Verification items for the finished model (mm, model axes). A direction names the side the tool comes from. Give positions to 0.01 mm unless a question says otherwise; leave off trailing zeros. Loops run counter-clockwise (first coordinate to the right, second up) from the corner with the lowest first, then second, coordinate; pieces in that order, holes last. Notation, with made-up numbers: M 45.5,53.25 L 81.5,53.25 A25 ccw 81.5,92.25 Z; hole C 46,61.5 d9. An arc over 180 degrees is marked long. Answer in a Markdown table with one row per item.
```python
from build123d import *

# Parameters (mm, degrees)
F0_W     = 45
F0_H     = 45
F1_DEPTH = 36
F2_T     = -2
F3_W     = 30
F3_H     = 30
F4_DEPTH = 25


with BuildPart() as f1:
    # F0 (on Front) → F1 (new body)
    with BuildSketch(Plane.XZ):
        Rectangle(F0_W, F0_H)
    extrude(amount=F1_DEPTH)

    # F2
    f2_openings = [f1.faces().sort_by_distance(p)[0] for p in [
        (0, -36, 0),
    ]]
    offset(amount=F2_T, openings=f2_openings)

    # F3 (on face) → F4 (cut)
    with BuildSketch(Plane(origin=(0, 0, 0), x_dir=(-1, 0, 0), z_dir=(0, 1, 0))):
        Rectangle(F3_W, F3_H)
    extrude(amount=-F4_DEPTH, mode=Mode.SUBTRACT)


solid = f1.part
```
Item 1: Sectioned sample at D-D (z = 19.5). Record the cut outline in (x, y).
Reported:
| item | result |
|---|---|
| outline | M -22.5,-36 L -20.5,-36 L -20.5,-2 L 20.5,-2 L 20.5,-36 L 22.5,-36 L 22.5,0 L -22.5,0 Z |
Item 2: Tool access check on faces 1 (the flat face through (0, -1, -15)), 2 (the flat face through (0, -19, -20.5)), 3 (the flat face through (-0.3, 0, 15.3)). Record the directions out of +Z, -Z, +X, -X, +Y, -Y that give a thin tool (end or side, any length) a straight path to the whole face; none if there is none.
Reported:
| item | result |
|---|---|
| face 1 | +Y, -Y |
| face 2 | -Y |
| face 3 | +Z, -Z, +X, -X, +Y |
Item 3: Sectioned sample at C-C (y = -8). Record the cut outline in (x, z).
Reported:
| item | result |
|---|---|
| outline | M -22.5,-22.5 L 22.5,-22.5 L 22.5,22.5 L -22.5,22.5 Z; hole M -20.5,-20.5 L 20.5,-20.5 L 20.5,20.5 L -20.5,20.5 Z |
Item 4: Sectioned sample at A-A (z = -13.5). Record the cut outline in (x, y), and give its area (3 significant figures).
Reported:
| item | result |
|---|---|
| outline | M -22.5,-36 L -20.5,-36 L -20.5,-2 L -15,-2 L -15,0 L -22.5,0 Z; M 15,-2 L 20.5,-2 L 20.5,-36 L 22.5,-36 L 22.5,0 L 15,0 Z |
| area | 166 mm^2 |
Item 5: Scan lines: L1, parallel to X at y = -12, z = -19; L2, parallel to Y at x = 14.5, z = 15.5. Record each from-to range of solid material in increasing order. Write a range as [from, to].
Reported:
| item | result |
|---|---|
| L1 | x = [-22.5, -20.5], [20.5, 22.5] |
| L2 | y = [-2, 0] |
Item 6: Release check for a two-part mould opening along Z. For faces 4 (the flat face through (22.5, -18, 0)), 5 (the flat face through (0, -18, -22.5)), 6 (the flat face through (-20.5, -19, 0)) record: released by +Z, released by -Z, zero draft, split by the parting line, or undercut.
Reported:
| item | result |
|---|---|
| face 4 | zero draft |
| face 5 | released by -Z |
| face 6 | undercut |
Item 7: Go/stop test with a flat-tipped pin: pin 1 (4 mm diameter, centred on x = -6, z = -16.5, fed in from -Y). Record where the tip stops, or that it passes through.
Reported:
| item | result |
|---|---|
| pin 1 | stops at y = -2 |
Item 8: Sectioned sample at B-B (x = -0.5). Record the cut outline in (y, z), and give its area (3 significant figures).
Reported:
| item | result |
|---|---|
| outline | M -36,-22.5 L 0,-22.5 L 0,-15 L -2,-15 L -2,-20.5 L -36,-20.5 Z; M -36,20.5 L -2,20.5 L -2,15 L 0,15 L 0,22.5 L -36,22.5 Z |
| area | 166 mm^2 |
